For this review, take the finished solid that the model builds, in its own axes (mm). A direction names the side the tool comes from. Coordinates: 2 decimals unless noted, no trailing zeros. Order: outer loops, then holes, each group sorted by start corner. A loop starts at its lowest first (then second) coordinate and runs counter-clockwise, first axis right, second up.
from build123d import *

# Parameters (mm, degrees)
SKETCH2_W   = 25.4
SKETCH2_H   = 25.4
SKETCH2_W_2 = 23
SKETCH2_H_2 = 23


with BuildPart() as part:
    # Sweep1: sweep along a path in Sketch1
    with BuildLine(Plane(origin=(0, 0, 0), x_dir=(1, 0, 0), z_dir=(0, 1, 0))) as sweep1_path:
        Line((-100, 605), (100, 605))
        Line((100, 605), (100, -605))
        Line((100, -605), (-100, -605))
        Line((-100, -605), (-100, 605))
    # Sketch2 → Sweep1 (sweep)
    with BuildSketch(Plane(origin=(0, 0, 0), x_dir=(0, 0, -1), z_dir=(1, 0, 0))):
        with Locations((-592.3, 12.7)):
            Rectangle(SKETCH2_W, SKETCH2_H)
        with Locations((-592.3, 12.7)):
            Rectangle(SKETCH2_W_2, SKETCH2_H_2, mode=Mode.SUBTRACT)
    sweep(path=sweep1_path.line, transition=Transition.RIGHT)


solid = part.part
1. Clearance check with a flat-ended pin moving along its axis: pin 1 Ø10 at (x, z) = (-66, 213.5) entering from +Y. State where the tip first meets the part, or that it passes through.
Answer below:
pin 1: passes through
2. The part is to be moulded in two halves that separate along X. For faces 1 (the face through (-100, 13, -8)), 2 (the face through (-1, 13, 605)), 3 (the face through (-80, 24.2, -92)), say which applies: +X half, -X half, draft (parallel to the pull), parting line (faces both ways), or undercut.
Answer below:
face 1: -X half
face 2: draft
face 3: undercut
3. To check wall thickness, follow L1, parallel to Z at x = 38.5, y = 19.75; L2, parallel to X at y = 10.5, z = -401.5; L3, parallel to Z at x = -83, y = 5.75. State the ranges of each line that lie inside material, in increasing order.
Answer below:
L1: z = -605 to -603.8, -580.8 to -579.6, 579.6 to 580.8, 603.8 to 605
L2: x = -100 to -98.8, -75.8 to -74.6, 74.6 to 75.8, 98.8 to 100
L3: z = -605 to -603.8, 603.8 to 605
4. Machinability: for faces 4 (the face through (-75.8, 13, -8)), 5 (the face through (1, 13, -605)), 6 (the face through (-74.6, 13, -8)), which of the approach directions +Z, -Z, +X, -X, +Y, -Y give a long, thin tool a straight path to every point of the face, cutting with its end or side? Answer none if there is none.
Answer below:
face 4: none
face 5: -Z, +X, -X, +Y, -Y
face 6: +Y, -Y
5. Take a section at B-B, the plane z = 270. Give the boundary of the cut face in (x, y).
Answer below:
outline: (-100, 0) - (-74.6, 0) - (-74.6, 25.4) - (-100, 25.4) - close; (74.6, 0) - (100, 0) - (100, 25.4) - (74.6, 25.4) - close; hole (-98.8, 1.2) - (-75.8, 1.2) - (-75.8, 24.2) - (-98.8, 24.2) - close; hole (75.8, 1.2) - (98.8, 1.2) - (98.8, 24.2) - (75.8, 24.2) - close
6. Take a section at A-A, the plane y = 6.25. Give the boundary of the cut face in (x, z).
Answer below:
outline: (-100, -605) - (100, -605) - (100, 605) - (-100, 605) - close; (-75.8, -580.8) - (75.8, -580.8) - (75.8, 580.8) - (-75.8, 580.8) - close; hole (-98.8, -603.8) - (98.8, -603.8) - (98.8, 603.8) - (-98.8, 603.8) - close; hole (-74.6, -579.6) - (74.6, -579.6) - (74.6, 579.6) - (-74.6, 579.6) - close
